Source: CAD feature listing. Evaluate the final solid. Frame: model axes, mm. Face numbers are marked on the shaded views. A direction names the side the tool comes from. Round coordinates to 2 decimals unless told otherwise and drop trailing zeros. Order: outer loops, then holes, each group sorted by start corner. A loop starts at its lowest first (then second) coordinate and runs counter-clockwise, first axis right, second up. Notation, with made-up numbers: (87.5, 66) -> (143.5, 66) arc R19 ccw to (143.5, 77) -> close; hole circle Ø5 at (23, 48.25). An arc over 180 degrees is marked (long way). Answer as CSV lines item,"result". Start each with the question number.
(1) Section query D-D (z = 4.75). Output: boundary loops of the cut face in (x, y).
(2) Set-up query: the marked faces 4 and 5. Return all of +Z, -Z, +X, -X, +Y, -Y with unobstructed straight access to the full face (end or side cutting, diameter ignored); none if empty.
(3) Contact query for flat-ended pins moving along their axis: P1, Ø3, axis at x = 9, z = 2, coming from the +Y side; P2, Ø2, axis at x = 1.5, z = -3, coming from the -Y side; P3, Ø1.5, axis at x = 10, y = -3.5, coming from the +Z side; P4, Ø5.5, axis at y = 0, z = 1, coming from the +X side. Output: stop coordinate, or through.
(4) Section query C-C (x = 5.25). Output: boundary loops of the cut face in (y, z).
(5) Section query B-B (y = 0.75). Output: boundary loops of the cut face in (x, z), plus the area to 3 significant figures.
(6) Section query A-A (z = 0). Output: boundary loops of the cut face in (x, y).
(7) Pull-direction query (Y, two-part tool) for the marked faces 1, 2 and 3; classes: +Y half, -Y half, draft (parallel to the pull), parting line (faces both ways), or undercut.
(8) Line query: line 1 along Y through (x, z) = (10.65, 0); line 2 along Y through (x, z) = (3.5, 0); line 3 along Z through (x, y) = (5.5, -2.5). Output: solid intervals per line, ascending. Write a range as from..to.
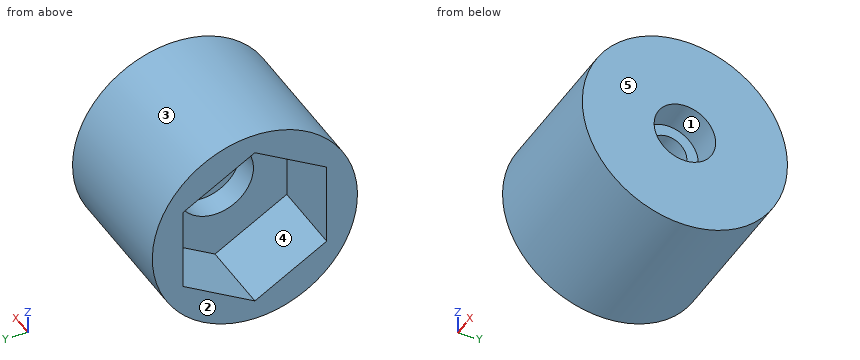
```python
from build123d import *

# Parameters (mm, degrees)
SKETCH1_R           = 8
BOSS_EXTRUDE1_DEPTH = 12
CUT_EXTRUDE1_DEPTH  = 6
SKETCH3_R           = 2.4
CUT_EXTRUDE2_DEPTH  = 2.6
SKETCH4_R           = 1.5
CUT_EXTRUDE3_DEPTH  = 10.4
SKETCH5_R           = 3
CUT_EXTRUDE4_DEPTH  = 2


with BuildPart() as part:
    # Sketch1 → Boss-Extrude1 (new body)
    with BuildSketch(Plane(origin=(0, 0, 0), x_dir=(0, 0, -1), z_dir=(1, 0, 0))):
        Circle(SKETCH1_R)
    extrude(amount=BOSS_EXTRUDE1_DEPTH)

    # Sketch2 → Cut-Extrude1 (cut)
    with BuildSketch(Plane.ZY):
        Polygon((6.466323015, 0), (3.233161507, 5.6), (-3.233161507, 5.6), (-6.466323015, 0), (-3.233161507, -5.6), (3.233161507, -5.6), align=None)
    extrude(amount=-CUT_EXTRUDE1_DEPTH, mode=Mode.SUBTRACT)

    # Sketch3 → Cut-Extrude2 (cut)
    with BuildSketch(Plane(origin=(12, 0, 0), x_dir=(0, 0, -1), z_dir=(1, 0, 0))):
        Circle(SKETCH3_R)
    extrude(amount=-CUT_EXTRUDE2_DEPTH, mode=Mode.SUBTRACT)

    # Sketch4 → Cut-Extrude3 (cut, through all)
    with BuildSketch(Plane(origin=(9.4, 0, 0), x_dir=(0, 0, -1), z_dir=(1, 0, 0))):
        Circle(SKETCH4_R)
    extrude(amount=-CUT_EXTRUDE3_DEPTH, mode=Mode.SUBTRACT)

    # Sketch5 → Cut-Extrude4 (cut)
    with BuildSketch(Plane.ZY.offset(-6)):
        Circle(SKETCH5_R)
    extrude(amount=-CUT_EXTRUDE4_DEPTH, mode=Mode.SUBTRACT)


solid = part.part
```
Answer block:
1,outline,"(0, -6.44) -> (12, -6.44) -> (12, 6.44) -> (0, 6.44) -> (0, 2.97) -> (6, 2.97) -> (6, -2.97) -> (0, -2.97) -> close"
2,face 4,"-X"
2,face 5,"+Z, -Z, +X, +Y, -Y"
3,P1,"y = 7.98"
3,P2,"y = -7.75"
3,P3,"z = 7.51"
3,P4,"x = 12"
4,outline,"circle Ø16 at (0, 0); hole (-5.6, -3.23) -> (0, -6.47) -> (5.6, -3.23) -> (5.6, 3.23) -> (0, 6.47) -> (-5.6, 3.23) -> close"
5,outline,"(0, -7.96) -> (12, -7.96) -> (12, -2.28) -> (9.4, -2.28) -> (9.4, -1.3) -> (8, -1.3) -> (8, -2.9) -> (6, -2.9) -> (6, -6.03) -> (0, -6.03) -> close; (0, 6.03) -> (6, 6.03) -> (6, 2.9) -> (8, 2.9) -> (8, 1.3) -> (9.4, 1.3) -> (9.4, 2.28) -> (12, 2.28) -> (12, 7.96) -> (0, 7.96) -> close"
5,area,"91.6 mm2"
6,outline,"(0, -8) -> (12, -8) -> (12, -2.4) -> (9.4, -2.4) -> (9.4, -1.5) -> (8, -1.5) -> (8, -3) -> (6, -3) -> (6, -5.6) -> (0, -5.6) -> close; (0, 5.6) -> (6, 5.6) -> (6, 3) -> (8, 3) -> (8, 1.5) -> (9.4, 1.5) -> (9.4, 2.4) -> (12, 2.4) -> (12, 8) -> (0, 8) -> close"
7,face 1,"undercut"
7,face 2,"draft"
7,face 3,"parting line"
8,line 1,"-8..-2.4, 2.4..8"
8,line 2,"-8..-5.6, 5.6..8"
8,line 3,"-7.6..-5.02, 5.02..7.6"
